Build history of the part. All positions in model axes, mm. A direction names the side the tool comes from. Give positions to 0.01 mm unless a question says otherwise; leave off trailing zeros. Write each loop counter-clockwise with the first axis right and the second up, starting at its lowest first coordinate (ties: lowest second). Pieces come first, ordered by that corner, then holes. Notation, with made-up numbers: (16.5, 51.5) -> (24.5, 51.5) arc R14 cw to (24.5, 71.5) -> close; hole circle Ø10 at (-16, 45). An arc over 180 degrees is marked (long way). One line per question, with ' | ' between items. Start each with the question number.
(1) Band-saw the part on A-A, the plane z = -15.5. Give the cut face in (x, y) (3 decimals), and give its area (3 significant figures).
(2) Tool access for faces 4 (the flat face through (14, 2.5, -15)), 5 (the flat face through (21.8, 0, 12.9)), 6 (the flat face through (8, -13, 9.95)), 7 (the flat face through (8.535, -2.652, -14.68)): list every direction of +Z, -Z, +X, -X, +Y, -Y with a clear straight run to the whole face (end or side of a thin tool).
(3) Drill centre lines: probe 1 along Y at (x, z) = (-22, -2); probe 2 along Z at (x, y) = (22.5, 2.1); probe 3 along X at (y, z) = (-2.5, 8). Where is each one in solid material? Low to high. Write a range as from..to.
(4) Band-saw the part on B-B, the plane z = 3.5. Give the cut face in (x, y), and give its area (3 significant figures).
(5) Pin check, flat tips, straight feed: P1, Ø12, axis at y = -14, z = -16, coming from the -X side; P2, Ø10, axis at y = -9.5, z = -15, coming from the +X side; P3, Ø3, axis at x = 22.5, z = 13.75, coming from the -Y side. Stop position of each tip, or through.
(6) Band-saw the part on D-D, the plane y = -8. Give the cut face in (x, z), and give its area (3 significant figures).
(7) Pull direction Y, two halves, no side cores. Call faces 1 (the cylindrical face through (-22, 1.5, -14.5)), 2 (the cylindrical face through (23.93, -16.9, -14.68)), 3 (the flat face through (13.284, -15.09, -14.68)): released by +Y, released by -Y, zero draft, split by the parting line, or undercut.
(8) Band-saw the part on C-C, the plane x = 1. Give the cut face in (y, z), and give its area (4 significant figures).
from build123d import *

# Parameters (mm, degrees)
SKETCH_1_R          = 0.9
EXTRUDE_1_DEPTH     = 3
EXTRUDE_2_DEPTH     = 19
EXTRUDE_3_DEPTH     = 2
SKETCH_5_W          = 8.7
SKETCH_5_H          = 4.7
CUT_EXTRUDE_1_DEPTH = 6.3
EXTRUDE_4_DEPTH     = 10


with BuildPart() as part:
    # 草图1 → 凸台-拉伸1 (new body)
    with BuildSketch(Plane(origin=(0, 0, 0), x_dir=(1, 0, 0), z_dir=(0, 1, 0))):
        with BuildLine():
            Line((4.5, 16.25), (4.5, 9.75))
            Line((4.5, 9.75), (25, 9.75))
            Line((25, 9.75), (25, -13.75))
            ThreePointArc((25, -13.75), (24.267766953, -15.517766953), (22.5, -16.25))
            Line((22.5, -16.25), (-20, -16.25))
            ThreePointArc((-20, -16.25), (-23.535533906, -14.785533906), (-25, -11.25))
            Line((-25, -11.25), (-25, 13.75))
            ThreePointArc((-25, 13.75), (-24.267766953, 15.517766953), (-22.5, 16.25))
            Line((-22.5, 16.25), (4.5, 16.25))
        make_face()
        with Locations((-22.5, 13.75)):
            Circle(SKETCH_1_R, mode=Mode.SUBTRACT)
        with Locations((22.5, -13.75)):
            Circle(SKETCH_1_R, mode=Mode.SUBTRACT)
    extrude(amount=EXTRUDE_1_DEPTH)

    # 草图2 → 凸台-拉伸2 (add)
    with BuildSketch(Plane(origin=(0, 3, 0), x_dir=(1, 0, 0), z_dir=(0, 1, 0))):
        with BuildLine():
            Line((4.5, 16.25), (-16.520869628, 16.25))
            ThreePointArc((-16.520869628, 16.25), (-18.55187923, 15.457940217), (-19.510434814, 13.5))
            ThreePointArc((-19.510434814, 13.5), (-20.378679656, 11.628679656), (-22.25, 10.760434814))
            ThreePointArc((-22.25, 10.760434814), (-24.207940217, 9.80187923), (-25, 7.770869628))
            Line((-25, 7.770869628), (-25, -11.25))
            ThreePointArc((-25, -11.25), (-23.535533906, -14.785533906), (-20, -16.25))
            Line((-20, -16.25), (16.520869628, -16.25))
            ThreePointArc((16.520869628, -16.25), (18.55187923, -15.457940217), (19.510434814, -13.5))
            ThreePointArc((19.510434814, -13.5), (20.378679656, -11.628679656), (22.25, -10.760434814))
            ThreePointArc((22.25, -10.760434814), (24.207940217, -9.80187923), (25, -7.770869628))
            Line((25, -7.770869628), (25, 9.75))
            Line((25, 9.75), (4.5, 9.75))
            Line((4.5, 9.75), (4.5, 16.25))
        make_face()
    extrude(amount=-EXTRUDE_2_DEPTH)

    # 草图4 → 凸台-拉伸3 (add)
    with BuildSketch(Plane.XZ.offset(16)):
        with BuildLine():
            Line((-0.7, -16.25), (-0.7, 16.25))
            Line((-0.7, 16.25), (16.520869628, 16.25))
            ThreePointArc((16.520869628, 16.25), (18.55187923, 15.457940217), (19.510434814, 13.5))
            ThreePointArc((19.510434814, 13.5), (20.378679656, 11.628679656), (22.25, 10.760434814))
            ThreePointArc((22.25, 10.760434814), (24.207940217, 9.80187923), (25, 7.770869628))
            Line((25, 7.770869628), (25, -9.75))
            Line((25, -9.75), (4.5, -9.75))
            Line((4.5, -9.75), (4.5, -16.25))
            Line((4.5, -16.25), (-0.7, -16.25))
        make_face()
    extrude(amount=EXTRUDE_3_DEPTH)

    # 草图5 → 切除-拉伸1 (cut)
    with BuildSketch(Plane.XY.offset(16.25)):
        with Locations((7.65, -13.25)):
            Rectangle(SKETCH_5_W, SKETCH_5_H)
    extrude(amount=-CUT_EXTRUDE_1_DEPTH, mode=Mode.SUBTRACT)

    # 草图6 → 凸台-拉伸4 (add)
    with BuildSketch(Plane(origin=(0, 0, -9.75), x_dir=(-1, 0, 0), z_dir=(0, 0, -1))):
        with BuildLine():
            Line((-6.5, 2.5), (-22.5, 2.5))
            ThreePointArc((-22.5, 2.5), (-23.914213562, 1.914213562), (-24.5, 0.5))
            Line((-24.5, 0.5), (-24.5, -15.5))
            ThreePointArc((-24.5, -15.5), (-23.914213562, -16.914213562), (-22.5, -17.5))
            Line((-22.5, -17.5), (-6.5, -17.5))
            ThreePointArc((-6.5, -17.5), (-5.085786438, -16.914213562), (-4.5, -15.5))
            Line((-4.5, -15.5), (-4.5, 0.5))
            ThreePointArc((-4.5, 0.5), (-5.085786438, 1.914213562), (-6.5, 2.5))
        make_face()
        with BuildLine():
            Line((-14.5, -13.75), (-12.034104017, -16.467126463))
            ThreePointArc((-12.034104017, -16.467126463), (-5.896292843, -11.030753907), (-6.445963745, -2.85))
            Line((-6.445963745, -2.85), (-8.548360144, -9.408004985))
            ThreePointArc((-8.548360144, -9.408004985), (-10.816423691, -12.549135132), (-14.5, -13.75))
        make_face(mode=Mode.SUBTRACT)
        with BuildLine():
            Line((-14.5, -16.8), (-19.128200716, -11.700268817))
            ThreePointArc((-19.128200716, -11.700268817), (-20.714467446, -8.165503094), (-19.912658774, -4.375))
            Line((-19.912658774, -4.375), (-23.498707307, -5.151965333))
            ThreePointArc((-23.498707307, -5.151965333), (-21.859576156, -13.185652012), (-14.5, -16.8))
        make_face(mode=Mode.SUBTRACT)
        with BuildLine():
            Line((-22.554036255, -2.85), (-15.823439141, -1.391726198))
            ThreePointArc((-15.823439141, -1.391726198), (-11.969108863, -1.785361774), (-9.087341226, -4.375))
            Line((-9.087341226, -4.375), (-7.967188676, -0.880908204))
            ThreePointArc((-7.967188676, -0.880908204), (-15.744131001, 1.716405918), (-22.554036255, -2.85))
        make_face(mode=Mode.SUBTRACT)
    extrude(amount=EXTRUDE_4_DEPTH)


solid = part.part
Results:
1) outline: (-24.285, 0) -> (-18.505, 0) -> (-18.505, -16) -> (-0.7, -16) -> (-0.7, -18) -> (4.5, -18) -> (4.5, -15.5) arc R2 ccw to (6.5, -17.5) -> (22.5, -17.5) arc R2 ccw to (24.5, -15.5) -> (24.5, 0.5) arc R2 ccw to (22.5, 2.5) -> (6.5, 2.5) arc R2 ccw to (4.5, 0.5) -> (4.5, 3) -> (-24.285, 3) -> close; hole (6.446, -2.85) arc R9.3 ccw to (12.034, -16.467) -> (14.5, -13.75) arc R6.25 cw to (8.548, -9.408) -> close; hole (7.967, -0.881) -> (9.087, -4.375) arc R6.25 cw to (15.823, -1.392) -> (22.554, -2.85) arc R9.3 ccw to start; hole (14.5, -16.8) arc R9.3 ccw to (23.499, -5.152) -> (19.913, -4.375) arc R6.25 cw to (19.128, -11.7) -> close | area: 740 mm²
2) face 4: -Z, +X, +Y | face 5: +Z, +X, -Y | face 6: +Z | face 7: -Z
3) probe 1: y = -16..3 | probe 2: z = -19.75..12.85, 14.65..16.25 | probe 3: x = -25..24.99
4) outline: (-25, -16) -> (-0.7, -16) -> (-0.7, -18) -> (25, -18) -> (25, 3) -> (-25, 3) -> close | area: 1,000 mm²
5) P1: stops at x = -24.01 | P2: stops at x = 24.5 | P3: stops at y = 0
6) outline: (-25, -7.77) arc R3 ccw to (-22.25, -10.76) arc R3 cw to (-19.51, -13.5) arc R3 ccw to (-16.52, -16.25) -> (4.5, -16.25) -> (4.5, -19.75) -> (5.21, -19.75) -> (5.21, -9.75) -> (8.1, -9.75) -> (8.1, -19.75) -> (20.73, -19.75) -> (20.73, -9.75) -> (23.79, -9.75) -> (23.79, -19.75) -> (24.5, -19.75) -> (24.5, -9.75) -> (25, -9.75) -> (25, 7.77) arc R3 ccw to (22.25, 10.76) arc R3 cw to (19.51, 13.5) arc R3 ccw to (16.52, 16.25) -> (-20, 16.25) arc R5 ccw to (-25, 11.25) -> close | area: 1,560 mm²
7) face 1: zero draft | face 2: released by -Y | face 3: undercut
8) outline: (-18, -16.25) -> (3, -16.25) -> (3, 16.25) -> (-18, 16.25) -> close | area: 682.5 mm²
